from build123d import *

# Parameters (mm, degrees)
SKETCH_1_W          = 32
SKETCH_1_H          = 24
EXTRUDE_1_DEPTH     = 1.2
SKETCH_2_W          = 23
SKETCH_2_H          = 24
EXTRUDE_2_DEPTH     = 5
SKETCH_6_W          = 32
SKETCH_6_H          = 5.5
EXTRUDE_5_DEPTH     = 9
SKETCH_8_R          = 1
CUT_EXTRUDE_7_DEPTH = 10


with BuildPart() as part:
    # 草图1 → 凸台-拉伸1 (new body)
    with BuildSketch(Plane(origin=(0, 0, 0), x_dir=(1, 0, 0), z_dir=(0, 1, 0))):
        Rectangle(SKETCH_1_W, SKETCH_1_H)
    extrude(amount=EXTRUDE_1_DEPTH)

    # 草图2 → 凸台-拉伸2 (add)
    with BuildSketch(Plane(origin=(0, 0, 0), x_dir=(1, 0, 0), z_dir=(0, 1, 0))):
        Rectangle(SKETCH_2_W, SKETCH_2_H)
    extrude(amount=EXTRUDE_2_DEPTH)

    # 草图5 → 旋转5 (revolve)
    with BuildSketch(Plane.XY):
        with BuildLine():
            Line((0, 5), (11.5, 5))
            ThreePointArc((11.5, 5), (8.131727984, 13.131727984), (0, 16.5))
            Line((0, 16.5), (0, 5))
        make_face()
    revolve(axis=Axis((0, 5, 0), (0, 1, 0)))

    # 草图6 → 凸台-拉伸5 (add)
    with BuildSketch(Plane(origin=(0, 0, 0), x_dir=(1, 0, 0), z_dir=(0, 1, 0))):
        with Locations((0, 9.25)):
            Rectangle(SKETCH_6_W, SKETCH_6_H)
        with Locations((0, -9.25)):
            Rectangle(SKETCH_6_W, SKETCH_6_H)
    extrude(amount=-EXTRUDE_5_DEPTH)

    # 草图8 → 切除-拉伸7 (cut)
    with BuildSketch(Plane(origin=(0, 0, 0), x_dir=(1, 0, 0), z_dir=(0, 1, 0))):
        with Locations((14.5, 0)):
            Circle(SKETCH_8_R)
        with Locations((-14.5, 0)):
            Circle(SKETCH_8_R)
    extrude(amount=CUT_EXTRUDE_7_DEPTH, mode=Mode.SUBTRACT)


solid = part.part
Geometry: final body of the model. Coordinates: model frame, mm. A direction names the side the tool comes from. Coordinates: 2 decimals unless noted, no trailing zeros. Order: outer loops, then holes, each group sorted by start corner. A loop starts at its lowest first (then second) coordinate and runs counter-clockwise, first axis right, second up.
(1) Section query D-D (x = 3). Return the cut outline in (y, z), plus the area to 3 significant figures.
(2) Section query A-A (y = -1.5). Return the cut outline in (x, z), plus the area to 3 significant figures.
(3) Material intervals for probe 1 along X at (y, z) = (0.65, 0); probe 2 along Z at (x, y) = (14.5, 0.85); probe 3 along Z at (x, y) = (-4, -1.75), sorted ascending.
(4) Section query B-B (x = -14.5). Return the cut outline in (y, z), plus the area to 3 significant figures.
(5) Section query C-C (z = 3.25). Return the cut outline in (x, y).
(6) First-contact query: pin 1 (1.8 mm diameter, centred on x = -14.5, z = 0, fed in from -Y) (3 decimals); pin 2 (4 mm diameter, centred on x = 11.5, z = 0, fed in from +Y); pin 3 (1.3 mm diameter, centred on x = 13, z = -2, fed in from +Y); pin 4 (3 mm diameter, centred on x = 14.5, z = 0, fed in from -Y). Flat tips, straight axial feed; report the tip coordinate or a pass-through.
(7) Draft query along Z for faces 5 (the face through (11.5, 3, 0)), 6 (the face through (15.454, 0.592, -0.3)), 7 (the face through (0, -2, -12)). Return one class per face: pulls with the +Z half, pulls with the -Z half, needs draft (parallel to the pull), parting line crosses it, or undercut.
(8) Access query for faces 1 (the face through (0, -4, 6.5)), 2 (the face through (-11.5, 3, 0)), 3 (the face through (-0.1, 5, 11.7)), 4 (the face through (-0.1, 5, -11.8)). Directions: +Z, -Z, +X, -X, +Y, -Y. A direction counts if a zero-diameter tool reaches every point of the face in a straight line with its end or side. Return the directions, or none.
Solution:
1. outline: (-9, -12) - (5, -12) - (5, -11.1) arc R11.1 ccw to (5, 11.1) - (5, 12) - (-9, 12) - (-9, 6.5) - (0, 6.5) - (0, -6.5) - (-9, -6.5) - close
1. area: 413 mm2
2. outline: (-16, -12) - (16, -12) - (16, -6.5) - (-16, -6.5) - close; (-16, 6.5) - (16, 6.5) - (16, 12) - (-16, 12) - close
2. area: 352 mm2
3. probe 1: x = -16 to -15.5, -13.5 to 13.5, 15.5 to 16
3. probe 2: z = -12 to -1, 1 to 12
3. probe 3: z = -12 to -6.5, 6.5 to 12
4. outline: (-9, -12) - (1.2, -12) - (1.2, -1) - (0, -1) - (0, -6.5) - (-9, -6.5) - close; (-9, 6.5) - (0, 6.5) - (0, 1) - (1.2, 1) - (1.2, 12) - (-9, 12) - close
4. area: 125 mm2
5. outline: (-16, 0) - (16, 0) - (16, 1.2) - (11.5, 1.2) - (11.5, 5) - (11.03, 5) arc R11.03 ccw to (-11.03, 5) - (-11.5, 5) - (-11.5, 1.2) - (-16, 1.2) - close
6. pin 1: passes through
6. pin 2: stops at y = 11.48
6. pin 3: stops at y = 1.2
6. pin 4: stops at y = 0
7. face 5: needs draft
7. face 6: undercut
7. face 7: pulls with the -Z half
8. face 1: +X, -X, -Y
8. face 2: +Z, -Z, -X, +Y
8. face 3: +Z, +Y
8. face 4: -Z, +Y
